Geometry: final body of the model. Coordinates: model frame, mm. A direction names the side the tool comes from. Round coordinates to 2 decimals unless told otherwise and drop trailing zeros. Write each loop counter-clockwise with the first axis right and the second up, starting at its lowest first coordinate (ties: lowest second). Pieces come first, ordered by that corner, then holes.
from build123d import *

# Parameters (mm, degrees)
SKETCH_1_R               = 42.5
EXTRUDE_1_DEPTH          = 25
SKETCH_2_OUTSIDE_W       = 111.556
SKETCH_2_OUTSIDE_H       = 111.556
SKETCH_2_OUTSIDE_R       = 32.5
CUT_EXTRUDE_1_DEPTH      = 21
PATTERN_CIRCULAR_1_COUNT = 8
SKETCH_5_R               = 10
CUT_EXTRUDE_2_DEPTH      = 2
PATTERN_CIRCULAR_2_COUNT = 6
FILLET_1_R               = 3


with BuildPart() as part:
    # 草图1 → 凸台-拉伸1 (new body)
    with BuildSketch(Plane.XY):
        Circle(SKETCH_1_R)
    extrude(amount=EXTRUDE_1_DEPTH)

    # 草图2 outside → 切除-拉伸1 (cut)
    with BuildSketch(Plane.XY.offset(25)):
        Rectangle(SKETCH_2_OUTSIDE_W, SKETCH_2_OUTSIDE_H)
        Circle(SKETCH_2_OUTSIDE_R, mode=Mode.SUBTRACT)
    extrude(amount=-CUT_EXTRUDE_1_DEPTH, mode=Mode.SUBTRACT)

    # 草图3 → 打孔尺寸(%根据)内六角圆柱头螺钉的类型1 (revolve, cut)
    with BuildSketch(Plane(origin=(0, 37.5, 4), x_dir=(0, -1, 0), z_dir=(1, 0, 0))):
        Polygon((0, 0), (0, 7.942065486), (2.4, 6.5), (2.4, 1), (4, 1), (4, 0), align=None)
    hole_wizard_1 = revolve(axis=Axis((0, 37.5, 10.35), (0, 0, -1)), mode=Mode.SUBTRACT)

    # 阵列(圆周)1: 打孔尺寸(%根据)内六角圆柱头螺钉的类型1 ×8 about axis
    pattern_circular_1_axis = Axis((0, 0, 0), (0, 0, 1))
    for i in range(1, PATTERN_CIRCULAR_1_COUNT):
        add(hole_wizard_1.rotate(pattern_circular_1_axis, i * 360 / PATTERN_CIRCULAR_1_COUNT), mode=Mode.SUBTRACT)

    # 草图5 → 切除-拉伸2 (cut)
    with BuildSketch(Plane.XY.offset(25)):
        Circle(SKETCH_5_R)
    extrude(amount=-CUT_EXTRUDE_2_DEPTH, mode=Mode.SUBTRACT)

    # 草图6 → M3 螺纹孔1 (revolve, cut)
    with BuildSketch(Plane(origin=(0, 22.5, 25), x_dir=(0, -1, 0), z_dir=(1, 0, 0))):
        Polygon((0, 0), (0, 7.251075774), (1.25, 6.5), (1.25, 0), align=None)
    hole_wizard_m3_1 = revolve(axis=Axis((0, 22.5, 31.35), (0, 0, -1)), mode=Mode.SUBTRACT)

    # 阵列(圆周)2: M3 螺纹孔1 ×6 about axis
    pattern_circular_2_axis = Axis((0, 0, 0), (0, 0, 1))
    for i in range(1, PATTERN_CIRCULAR_2_COUNT):
        add(hole_wizard_m3_1.rotate(pattern_circular_2_axis, i * 360 / PATTERN_CIRCULAR_2_COUNT), mode=Mode.SUBTRACT)

    # 圆角1
    fillet_1_edges = [part.edges().sort_by_distance(p)[0] for p in [
        (-32.5, 0, 25),
    ]]
    fillet(fillet_1_edges, radius=FILLET_1_R)


solid = part.part
1) Draft query along X for faces 3 (the flat face through (12, -31, 4)), 4 (the cylindrical face through (-41.496, -0.176, 3.507)). Return one class per face: pulls with the +X half, pulls with the -X half, needs draft (parallel to the pull), parting line crosses it, or undercut.
2) Reachability of faces 1 (the cylindrical face through (22.82, -24.99, 3.51)), 2 (the cylindrical face through (28.914, -26.62, 1.521)) from +Z, -Z, +X, -X, +Y, -Y: full face, straight path, thin tool, end or side. Return the list, or none.
3) Section A-A on y = -37.5. Output: boundary loops of the cut face in (x, z).
4) Line query: probe 1 along X at (y, z) = (37.5, 3.35); probe 2 along Z at (x, y) = (30.5, -14); probe 3 along X at (y, z) = (37.5, 1.5). Output: solid intervals per line, ascending.
5) First-contact query: P1, Ø2.5, axis at x = 26.5, y = -28, coming from the +Z side; P2, Ø2, axis at y = -7, z = 10.5, coming from the +X side; P3, Ø6.5, axis at x = -38, y = -2, coming from the +Z side. Flat tips, straight axial feed; report the tip coordinate or a pass-through.
6) Section C-C on y = 0. State how many separate pieces and enclosed holes the cut face has, plus the area to 3 significant figures.
7) Section D-D on z = 16. Output: boundary loops of the cut face in (x, y), plus the area to 3 significant figures.
Filled in:
1. face 3: needs draft
1. face 4: undercut
2. face 1: +Z
2. face 2: +Z, -Z
3. outline: (-20, 0) - (-2.4, 0) - (-2.4, 3) - (-4, 3) - (-4, 4) - (-20, 4) - close; (2.4, 0) - (20, 0) - (20, 4) - (4, 4) - (4, 3) - (2.4, 3) - close
4. probe 1: x = -20 to -4, 4 to 20
4. probe 2: z = 0 to 4
4. probe 3: x = -20 to -2.4, 2.4 to 20
5. P1: stops at z = 3
5. P2: stops at x = 31.94
5. P3: stops at z = 4
6. separate pieces: 3
6. enclosed holes: 0
6. area: 1,620 mm2
7. outline: circle Ø65 at (0, 0)
7. area: 3,320 mm2
